Work out the finished part from the listing and answer in its coordinate system (mm). Round coordinates to 2 decimals unless told otherwise and drop trailing zeros. Order: outer loops, then holes, each group sorted by start corner. A loop starts at its lowest first (then second) coordinate and runs counter-clockwise, first axis right, second up.
Autodesk Inventor part; units mm, degrees
ref_plane "Start Plane" through (0, 0, 0) normal (0, 0, 1) x (1, 0, 0)
ref_plane "End Plane" through (0, 0, 304.8) normal (0, 0, 1) x (1, 0, 0)
ref_plane "YZ Plane" through (0, 0, 0) normal (1, 0, 0) x (0, 1, 0)
ref_plane "Start Plane" through (0, 0, 0) normal (0, 0, 1) x (1, 0, 0)
ref_plane "End Plane" through (0, 0, 304.8) normal (0, 0, 1) x (1, 0, 0)
sketch "Sketch" plane through (0, 0, 0) normal (0, 0, 1) x (1, 0, 0)
  arc A0 (-11.6332, 12.7) -> (-12.7, 11.6332) centre (-11.6332, 11.6332) ccw
  arc A1 (-5.3594, 10.5664) -> (-5.3594, 12.7) centre (-5.3594, 11.6332) ccw
  arc A2 (-12.7, 5.3594) -> (-10.5664, 5.3594) centre (-11.6332, 5.3594) ccw
  line L0 (-10.5664, 7.493) -> (-10.5664, 5.3594)
  line L1 (-7.493, 10.5664) -> (-5.3594, 10.5664)
  arc A3 (-9.6992, 7.8522) -> (-10.5664, 7.493) centre (-10.0584, 7.493) ccw
  arc A4 (-7.493, 10.5664) -> (-7.8522, 9.6992) centre (-7.493, 10.0584) ccw
  line L2 (-11.6332, 11.6332) -> (0, 0) construction
  line L3 (-5.8003, 3.9533) -> (-9.6992, 7.8522)
  line L4 (-7.8522, 9.6992) -> (-3.9533, 5.8003)
  arc A5 (-3.9533, 5.8003) -> (-2.6924, 5.278) centre (-2.6924, 7.0612) ccw
  arc A6 (-5.278, 2.6924) -> (-5.8003, 3.9533) centre (-7.0612, 2.6924) ccw
  arc A7 (0, 2.54) -> (-2.54, 0) centre (0, 0) ccw construction
  line L5 (0, 0) -> (-12.7, 0) construction
  line L6 (0, 12.7) -> (0, 0) construction
  arc A8 (-11.6332, 12.7) -> (-10.6172, 12.7) centre (-11.1252, 12.7) ccw
  arc A9 (-7.5692, 12.7) -> (-6.5532, 12.7) centre (-7.0612, 12.7) ccw
  arc A10 (-12.7, 10.6172) -> (-12.7, 11.6332) centre (-12.7, 11.1252) ccw
  arc A11 (-12.7, 6.5532) -> (-12.7, 7.5692) centre (-12.7, 7.0612) ccw
  line L7 (-12.7, 10.6172) -> (-12.7, 7.5692)
  line L8 (-12.7, 6.5532) -> (-12.7, 5.3594)
  line L9 (-10.6172, 12.7) -> (-7.5692, 12.7)
  line L10 (-6.5532, 12.7) -> (-5.3594, 12.7)
  circle A12 centre (0, 0) radius 2.54
  arc A13 (-12.7, -11.6332) -> (-11.6332, -12.7) centre (-11.6332, -11.6332) ccw
  line L11 (-12.7, -10.6172) -> (-12.7, -7.5692)
  arc A14 (-10.5664, -7.493) -> (-9.6992, -7.8522) centre (-10.0584, -7.493) ccw
  line L12 (-9.6992, -7.8522) -> (-5.8003, -3.9533)
  line L13 (-11.6332, -11.6332) -> (0, 0) construction
  line L14 (-3.9533, -5.8003) -> (-7.8522, -9.6992)
  arc A15 (-7.8522, -9.6992) -> (-7.493, -10.5664) centre (-7.493, -10.0584) ccw
  line L15 (-10.6172, -12.7) -> (-7.5692, -12.7)
  line L16 (-7.493, -10.5664) -> (-5.3594, -10.5664)
  arc A16 (-6.5532, -12.7) -> (-7.5692, -12.7) centre (-7.0612, -12.7) ccw
  line L17 (-6.5532, -12.7) -> (-5.3594, -12.7)
  arc A17 (-5.3594, -12.7) -> (-5.3594, -10.5664) centre (-5.3594, -11.6332) ccw
  arc A18 (-10.6172, -12.7) -> (-11.6332, -12.7) centre (-11.1252, -12.7) ccw
  arc A19 (-12.7, -11.6332) -> (-12.7, -10.6172) centre (-12.7, -11.1252) ccw
  arc A20 (-2.6924, -5.278) -> (-3.9533, -5.8003) centre (-2.6924, -7.0612) ccw
  arc A21 (-5.8003, -3.9533) -> (-5.278, -2.6924) centre (-7.0612, -2.6924) ccw
  line L18 (-10.5664, -7.493) -> (-10.5664, -5.3594)
  line L19 (-12.7, -6.5532) -> (-12.7, -5.3594)
  arc A22 (-10.5664, -5.3594) -> (-12.7, -5.3594) centre (-11.6332, -5.3594) ccw
  arc A23 (-12.7, -7.5692) -> (-12.7, -6.5532) centre (-12.7, -7.0612) ccw
  arc A24 (11.6332, -12.7) -> (12.7, -11.6332) centre (11.6332, -11.6332) ccw
  line L20 (10.6172, -12.7) -> (7.5692, -12.7)
  arc A25 (7.493, -10.5664) -> (7.8522, -9.6992) centre (7.493, -10.0584) ccw
  line L21 (7.8522, -9.6992) -> (3.9533, -5.8003)
  line L22 (11.6332, -11.6332) -> (0, 0) construction
  line L23 (5.8003, -3.9533) -> (9.6992, -7.8522)
  arc A26 (9.6992, -7.8522) -> (10.5664, -7.493) centre (10.0584, -7.493) ccw
  line L24 (12.7, -10.6172) -> (12.7, -7.5692)
  line L25 (10.5664, -7.493) -> (10.5664, -5.3594)
  arc A27 (12.7, -6.5532) -> (12.7, -7.5692) centre (12.7, -7.0612) ccw
  line L26 (12.7, -6.5532) -> (12.7, -5.3594)
  arc A28 (12.7, -5.3594) -> (10.5664, -5.3594) centre (11.6332, -5.3594) ccw
  arc A29 (12.7, -10.6172) -> (12.7, -11.6332) centre (12.7, -11.1252) ccw
  arc A30 (11.6332, -12.7) -> (10.6172, -12.7) centre (11.1252, -12.7) ccw
  arc A31 (5.278, -2.6924) -> (5.8003, -3.9533) centre (7.0612, -2.6924) ccw
  arc A32 (3.9533, -5.8003) -> (2.6924, -5.278) centre (2.6924, -7.0612) ccw
  line L27 (7.493, -10.5664) -> (5.3594, -10.5664)
  line L28 (6.5532, -12.7) -> (5.3594, -12.7)
  arc A33 (5.3594, -10.5664) -> (5.3594, -12.7) centre (5.3594, -11.6332) ccw
  arc A34 (7.5692, -12.7) -> (6.5532, -12.7) centre (7.0612, -12.7) ccw
  arc A35 (12.7, 11.6332) -> (11.6332, 12.7) centre (11.6332, 11.6332) ccw
  line L29 (12.7, 10.6172) -> (12.7, 7.5692)
  arc A36 (10.5664, 7.493) -> (9.6992, 7.8522) centre (10.0584, 7.493) ccw
  line L30 (9.6992, 7.8522) -> (5.8003, 3.9533)
  line L31 (11.6332, 11.6332) -> (0, 0) construction
  line L32 (3.9533, 5.8003) -> (7.8522, 9.6992)
  arc A37 (7.8522, 9.6992) -> (7.493, 10.5664) centre (7.493, 10.0584) ccw
  line L33 (10.6172, 12.7) -> (7.5692, 12.7)
  line L34 (7.493, 10.5664) -> (5.3594, 10.5664)
  arc A38 (6.5532, 12.7) -> (7.5692, 12.7) centre (7.0612, 12.7) ccw
  line L35 (6.5532, 12.7) -> (5.3594, 12.7)
  arc A39 (5.3594, 12.7) -> (5.3594, 10.5664) centre (5.3594, 11.6332) ccw
  arc A40 (10.6172, 12.7) -> (11.6332, 12.7) centre (11.1252, 12.7) ccw
  arc A41 (12.7, 11.6332) -> (12.7, 10.6172) centre (12.7, 11.1252) ccw
  arc A42 (2.6924, 5.278) -> (3.9533, 5.8003) centre (2.6924, 7.0612) ccw
  arc A43 (5.8003, 3.9533) -> (5.278, 2.6924) centre (7.0612, 2.6924) ccw
  line L36 (10.5664, 7.493) -> (10.5664, 5.3594)
  line L37 (12.7, 6.5532) -> (12.7, 5.3594)
  arc A44 (10.5664, 5.3594) -> (12.7, 5.3594) centre (11.6332, 5.3594) ccw
  arc A45 (12.7, 7.5692) -> (12.7, 6.5532) centre (12.7, 7.0612) ccw
  line L38 (-2.6924, 5.278) -> (2.6924, 5.278)
  line L39 (-5.278, 2.6924) -> (-5.278, -2.6924)
  line L40 (-2.6924, -5.278) -> (2.6924, -5.278)
  line L41 (5.278, -2.6924) -> (5.278, 2.6924)
  point P0 (0, 0)
  point P1 (0, 0)
  dimension "d2" = 2.1336
  dimension "d3" = 6.2738
  dimension "d4" = 6.2738
  dimension "d5" = 1.0668
  dimension "d6" = 2.1336
  dimension "d7" = 2.1336
  dimension "d8" = 1.016
  dimension "d9" = 1.016
  dimension "d10" = 135
  dimension "d11" = 2.667
  dimension "d12" = 4.572
  dimension "d13" = 4.572
  dimension "d14" = 2.667
  dimension "d15" = 5.08
  dimension "d16" = 45
  dimension "d19" = 45
  dimension "d20" = 0.508
  dimension "d21" = 4.572
  dimension "d22" = 1.016
  dimension "d23" = 4.572
  dimension "d24" = 1.016
  dimension "d25" = 0.508
  dimension "d26" = 0.508
  dimension "d27" = 0.508
  dimension "d28" = 12.7
  dimension "d37" = 360
  dimension "d47" = 10.5664
  dimension "d48" = 12.7
extrude "Body" add sketch "Sketch" along normal up to surface (304.8 mm away) from surface at 0
sketch "Sketch2" plane through (0, 0, 0) normal (0, 0, 1) x (1, 0, 0)
  line L0 (0, 0) -> (10, 0)
ref_plane "Work Plane3" through (0, 0, 0) normal (0, -1, 0) x (1, 0, 0)
sketch "Sketch3" plane through (0, 0, 0) normal (0, -1, 0) x (1, 0, 0)
  line L0 (-2, 0) -> (12, 0)
  line L1 (-2, 304.8) -> (12, 304.8)
  dimension "d60" = 304.8
equation "\"d3\" = d4"
equation "\"d6\" = d7"
equation "\"d11\" = d14"
equation "\"d12\" = d13"
equation "\"d23\" = d21"
equation "\"d24\" = d30"
equation "\"d26\" = 0.5 * d24"
equation "\"d27\" = 0.5 * d22"
equation "\"Width\" = 2 * d28"
equation "\"Height\" = 2 * d48"
equation "\"G_OFFSET_START\" = 0"
equation "\"G_OFFSET_END\" = 0"
equation "\"d56\" = Length + G_OFFSET_END"
equation "\"G_L\" = 304.8"
properties part number "1010_80_20" material "Aluminum-6061"
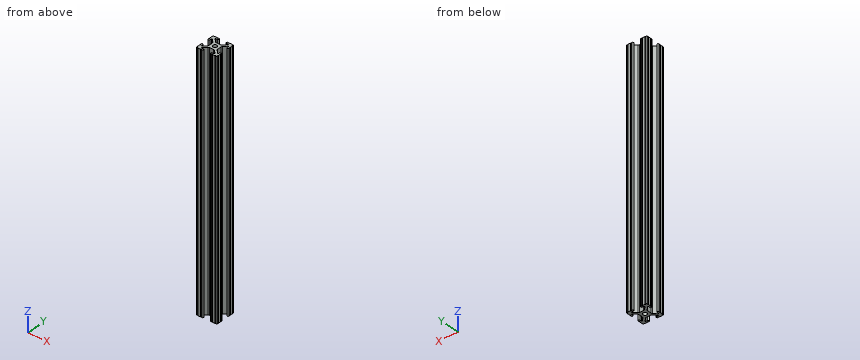
Item 1: Find section A-A (x = 0). Write down the section's boundary in (y, z), plus the area to 3 significant figures.
Item 2: Given pin 1 (4.5 mm diameter, centred on x = 0.5, z = 195.5, fed in from +Y); pin 2 (1.6 mm diameter, centred on x = 0.5, z = 130.5, fed in from -Y); pin 3 (6 mm diameter, centred on y = 1, z = 194.5, fed in from -X), each flat-ended and moving along its own axis, determine where each tip first touches the part or whether it passes through.
Item 3: Find the intervals of material crossed by line 1 along Y through (x, z) = (7.5, 218); line 2 along X through (y, z) = (-4.75, 31.5); line 3 along Y through (x, z) = (0, 179), in increasing order.
Model answer:
1. outline: (-5.28, 0) - (-2.54, 0) - (-2.54, 304.8) - (-5.28, 304.8) - close; (2.54, 0) - (5.28, 0) - (5.28, 304.8) - (2.54, 304.8) - close
1. area: 1,670 mm2
2. pin 1: stops at y = 5.28
2. pin 2: stops at y = -5.28
2. pin 3: stops at x = -5.85
3. line 1: y = -12.44 to -10.57, -9.35 to -5.65, 5.65 to 9.35, 10.57 to 12.44
3. line 2: x = -12.51 to -10.76, -6.6 to 6.6, 10.76 to 12.51
3. line 3: y = -5.28 to -2.54, 2.54 to 5.28
